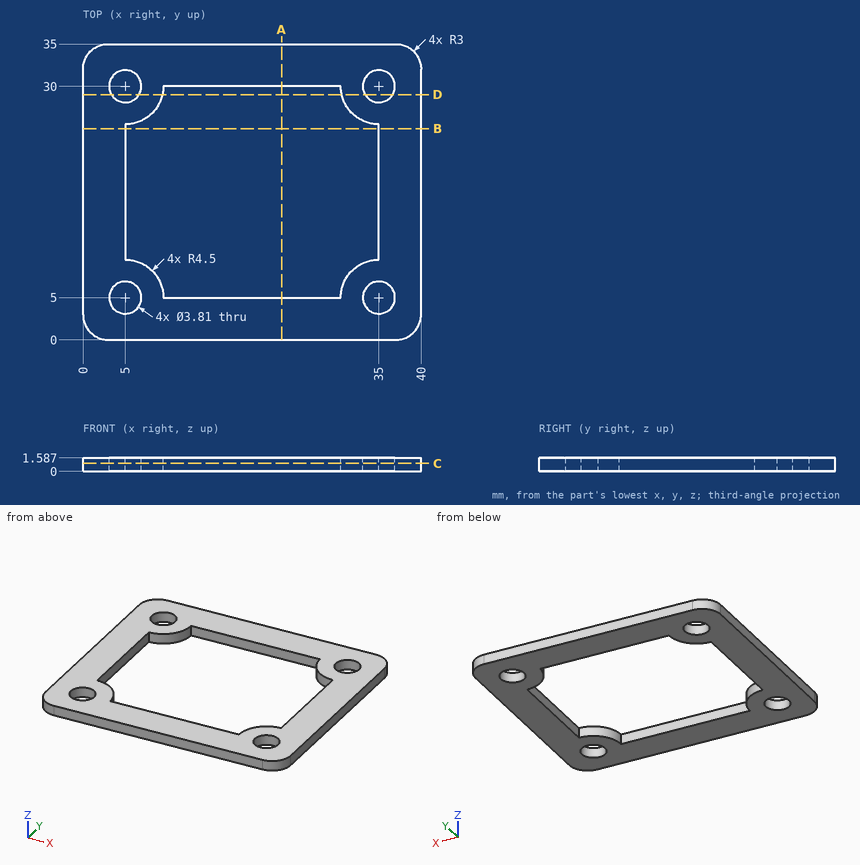
Input: dimensioned drawing with shaded views. Units: mm. Origin: part minimum x, y, z. Give positions to 0.01 mm unless a question says otherwise; leave off trailing zeros. Write each loop counter-clockwise with the first axis right and the second up, starting at its lowest first coordinate (ties: lowest second). Pieces come first, ordered by that corner, then holes. Notation, with made-up numbers: M 32,2 L 84,2 A35 ccw 84,36 Z; hole C 58,38 d10. An arc over 180 degrees is marked long. Write item = value, one per line. Start each with the question number.
1) Cut plane A-A on x = 23.5. Return the cut outline in (y, z).
2) Cut plane D-D on y = 29. Return the cut outline in (x, z).
3) First-contact query: pin 1 Ø0.5 at (x, z) = (15.5, 0.5) entering from -Y. Flat tip, straight axial feed; report the tip coordinate or a pass-through.
4) Cut plane C-C on z = 0.95. Return the cut outline in (x, y) (1 decimal).
5) Material intervals for line 1 along Y through (x, z) = (30, 1.1); line 2 along X through (y, z) = (21, 1); line 3 along Y through (x, z) = (34.5, 0.55), sorted ascending. Write a range as [from, to].
6) Cut plane B-B on y = 25. Return the cut outline in (x, z).
Solved:
q1.outline = M 0,0 L 5,0 L 5,1.59 L 0,1.59 Z; M 30,0 L 35,0 L 35,1.59 L 30,1.59 Z
q2.outline = M 0,0 L 3.38,0 L 3.38,1.59 L 0,1.59 Z; M 6.62,0 L 9.39,0 L 9.39,1.59 L 6.62,1.59 Z; M 30.61,0 L 33.38,0 L 33.38,1.59 L 30.61,1.59 Z; M 36.62,0 L 40,0 L 40,1.59 L 36.62,1.59 Z
q3.pin_1 = 0
q4.outline = M 0,3 A3 ccw 3,0 L 37,0 A3 ccw 40,3 L 40,32 A3 ccw 37,35 L 3,35 A3 ccw 0,32 Z; hole C 5,5 d3.8; hole C 5,30 d3.8; hole M 5,9.5 A4.5 cw 9.5,5 L 30.5,5 A4.5 cw 35,9.5 L 35,25.5 A4.5 cw 30.5,30 L 9.5,30 A4.5 cw 5,25.5 Z; hole C 35,5 d3.8; hole C 35,30 d3.8
q5.line_1 = [0, 5], [30, 35]
q5.line_2 = [0, 5], [35, 40]
q5.line_3 = [0, 3.16], [6.84, 9.47], [25.53, 28.16], [31.84, 35]
q6.outline = M 0,0 L 5,0 L 5,1.59 L 0,1.59 Z; M 35,0 L 40,0 L 40,1.59 L 35,1.59 Z
